Check sheet for the drawn part. Datum: minimum x, y, z corner. Units: mm. Round coordinates to 2 decimals unless told otherwise and drop trailing zeros. Write each loop counter-clockwise with the first axis right and the second up, starting at its lowest first coordinate (ties: lowest second). Pieces come first, ordered by that corner, then holes. Notation, with made-up numbers: (-5.75, 47) - (46.25, 47) arc R31 cw to (46.25, 72) - close; hole circle Ø8 at (7, -20). An arc over 180 degrees is marked (long way). Answer as a JSON object with one key per item and string values. Group by question number.
1) Thickness scan on line 1 (Z direction, x = 193, y = 50.5); line 2 (Y direction, x = 60, z = 111.5); line 3 (Y direction, x = 9, z = 152.5). Record the ranges inside material, lowest first.
2) Go/stop test with a flat-tipped pin: pin 1 Ø10 at (x, z) = (202.5, 175.5) entering from -Y. Record where the tip stops, or that it passes through.
3) Section check C-C (x = 104.5). Enter the section's corners in (y, z), then the cut area to 3 significant figures.
4) Section check B-B (y = 258). Enter the section's corners in (x, z).
5) Mould release check, pull along Y, two halves, no side actions. Record for the marked faces 1 and 2: +Y half, -Y half, draft (parallel to the pull), parting line (faces both ways), or undercut.
6) Section check A-A (z = 221). Enter the section's corners in (x, y).
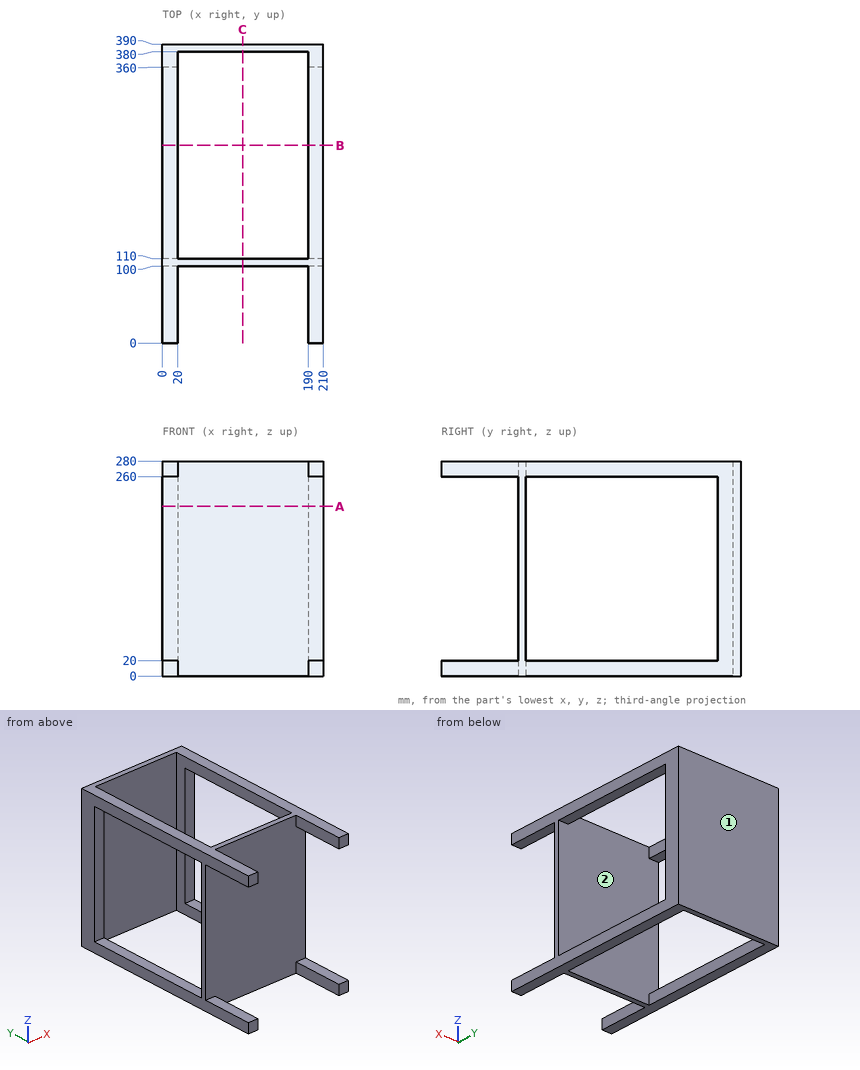
Returned:
{
 "1": {"line 1": "0 to 20, 260 to 280", "line 2": "100 to 110, 380 to 390", "line 3": "100 to 110, 360 to 390"},
 "2": {"pin 1": "y = 100"},
 "3": {"outline": "(100, 0) - (110, 0) - (110, 280) - (100, 280) - close; (380, 0) - (390, 0) - (390, 280) - (380, 280) - close", "area": "5,600 mm2"},
 "4": {"outline": "(0, 0) - (20, 0) - (20, 20) - (0, 20) - close; (0, 260) - (20, 260) - (20, 280) - (0, 280) - close; (190, 0) - (210, 0) - (210, 20) - (190, 20) - close; (190, 260) - (210, 260) - (210, 280) - (190, 280) - close"},
 "5": {"face 1": "+Y half", "face 2": "undercut"},
 "6": {"outline": "(0, 100) - (210, 100) - (210, 110) - (0, 110) - close; (0, 360) - (20, 360) - (20, 380) - (190, 380) - (190, 360) - (210, 360) - (210, 390) - (0, 390) - close"}
}
